Model file for the job. Use its own axes, mm. Face numbers are marked on the shaded views. Coordinates: 2 decimals unless noted, no trailing zeros. Use one line per item in the form item = value.
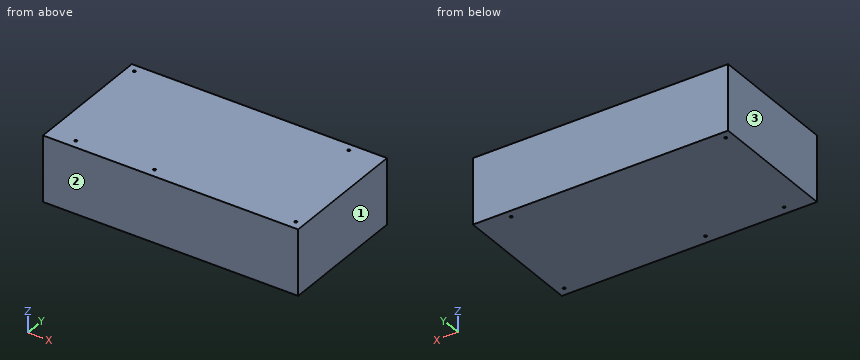
```python
from build123d import *

# Parameters (mm, degrees)
SKETCH1_W                   = 247
SKETCH1_H                   = 127
BOSS_EXTRUDE1_DEPTH         = 63.5
F_41_0_096_DIAMETER_HOLE1_D = 2.4384


with BuildPart() as part:
    # Sketch1 → Boss-Extrude1 (new body)
    with BuildSketch(Plane.XY):
        Rectangle(SKETCH1_W, SKETCH1_H)
    extrude(amount=BOSS_EXTRUDE1_DEPTH)

    # #41 (0.096) Diameter Hole1 (through all)
    with Locations(Plane.XY.offset(63.5)):
        with Locations((-115.88, 55.88), (-97.465, -55.118), (-21.265, -55.118), (115.641, -55.118), (91.7015, 55.88)):
            Hole(F_41_0_096_DIAMETER_HOLE1_D / 2)


solid = part.part
```
Q1. Wall check: line 1 along X through (y, z) = (56, 19); line 2 along X through (y, z) = (55, 33); line 3 along Y through (x, z) = (-115, 25). Give the ranges that are in metal, low to high.
Result:
line_1 = -123.5 to -117.09, -114.67 to 90.49, 92.91 to 123.5
line_2 = -123.5 to -116.72, -115.04 to 90.86, 92.55 to 123.5
line_3 = -63.5 to 55.04, 56.72 to 63.5
Q2. Mould opens along X. For the marked faces 1, 2 and 3 say: released by +X, released by -X, zero draft, split by the parting line, or undercut.
Result:
face_1 = released by +X
face_2 = zero draft
face_3 = released by -X
Q3. Pin check, flat tip, straight feed: pin 1 Ø1.5 at (x, y) = (91.7, 55.88) entering from -Z. Stop position of the tip, or through.
Result:
pin_1 = through
